Autodesk Inventor part; units mm, degrees
ref_plane "YZ Plane" through (0, 0, 0) normal (1, 0, 0) x (0, 1, 0)
ref_plane "XZ Plane" through (0, 0, 0) normal (0, 1, 0) x (-1, 0, 0)
ref_plane "XY Plane" through (0, 0, 0) normal (0, 0, 1) x (1, 0, 0)
sketch "Sketch1" plane through (0, 0, 0) normal (0, 1, 0) x (-1, 0, 0)
  circle A0 centre (4.364, -12.8492) radius 1.25
  line L0 (2.1213, -19.0919) -> (-8.4853, -8.4853)
  line L1 (10.6066, -10.6066) -> (0, 0)
  line L2 (0, 0) -> (-8.4853, -8.4853)
  circle A1 centre (-0.7071, -7.7782) radius 1.25
  line L3 (2.1213, -19.0919) -> (41.8977, -58.8682)
  line L4 (10.6066, -10.6066) -> (50.383, -50.383)
  arc A2 (41.8977, -58.8682) -> (50.383, -50.383) centre (55.8614, -64.3467) ccw
  circle A3 centre (62.579, -71.0642) radius 1.5
  circle A4 centre (49.1439, -57.6292) radius 1.5
  circle A5 centre (50.2046, -70.0036) radius 1.5
  circle A6 centre (61.5183, -58.6899) radius 1.5
  point P0 (0, 0)
  dimension "d3" = 3
  dimension "d4" = 3
  dimension "d5" = 3
  dimension "d6" = 3
extrude "Extrusion1" add sketch "Sketch1" along normal blind 3
sketch "Sketch2" plane through (0, 3, 0) normal (0, 1, 0) x (1, 0, 0)
  arc A0 (-41.8977, 58.8682) -> (-50.383, 50.383) centre (-55.8614, 64.3467) ccw
  circle A1 centre (-55.8614, 64.3467) radius 4
  point P0 (0, 0)
  dimension "d9" = 8
extrude "Extrusion2" cut sketch "Sketch2" against normal blind 3
properties part number "arm"
For this review, take the finished solid that the model builds, in its own axes (mm). Round coordinates to 2 decimals unless told otherwise and drop trailing zeros. Order: outer loops, then holes, each group sorted by start corner. A loop starts at its lowest first (then second) coordinate and runs counter-clockwise, first axis right, second up. Notation, with made-up numbers: (-20, 89) -> (-5, 89) arc R35 cw to (-5, 126) -> close; hole circle Ø3 at (59.25, 40). An arc over 180 degrees is marked (long way). Put each result on its own line as item: value.
Q1. Mouldability with a two-part tool opening along X and no side actions: class faces 1 (the cylindrical face through (0.13, 1.48, -6.67)), 2 (the flat face through (4, 1, -4)), 3 (the flat face through (-37, 3, -45)) as pulls with the +X half, pulls with the -X half, needs draft (parallel to the pull), parting line crosses it, or undercut.
Check result:
face 1: undercut
face 2: pulls with the +X half
face 3: needs draft
Q2. Insertion check: pin 1 Ø1.5 at (x, z) = (-4.36, -12.85) entering from +Y. The pin has a flat end and moves straight along its axis. Give the tip position at first contact, or say it passes through.
Check result:
pin 1: through
Q3. For probe 1 along Z at (x, y) = (-56, 0.25); probe 2 along Z at (x, y) = (-50, 2.8); probe 3 along Z at (x, y) = (-62, 0.75), list the stretches that pass through material, from the lowest coordinate up. Write a range as [from, to].
Check result:
probe 1: [-79.35, -68.34], [-60.35, -49.35]
probe 2: [-78.15, -71.49], [-68.52, -58.86], [-56.4, -50]
probe 3: [-78.03, -72.45], [-69.68, -60.11], [-57.27, -50.66]
Q4. Add section B-B on y = 1.6. Write out the cut boundary in (x, z), plus the area to 3 significant figures.
Check result:
outline: (-50.38, -50.38) arc R15 ccw (long way) to (-41.9, -58.87) -> (-2.12, -19.09) -> (8.49, -8.49) -> (0, 0) -> close; hole circle Ø3 at (-62.58, -71.06); hole circle Ø3 at (-61.52, -58.69); hole circle Ø8 at (-55.86, -64.35); hole circle Ø3 at (-50.2, -70); hole circle Ø3 at (-49.14, -57.63); hole circle Ø2.5 at (-4.36, -12.85); hole circle Ø2.5 at (0.71, -7.78)
area: 1,460 mm2
Q5. Add section C-C on x = -65. Write out the cut boundary in (y, z), plus the area to 3 significant figures.
Check result:
outline: (0, -76.24) -> (3, -76.24) -> (3, -52.45) -> (0, -52.45) -> close
area: 71.4 mm2
Q6. Add section D-D on z = -22. Write out the cut boundary in (x, y).
Check result:
outline: (-22, 0) -> (-5.03, 0) -> (-5.03, 3) -> (-22, 3) -> close
Q7. Add section A-A on x = -55.5. Write out the cut boundary in (y, z).
Check result:
outline: (0, -79.34) -> (3, -79.34) -> (3, -68.33) -> (0, -68.33) -> close; (0, -60.36) -> (3, -60.36) -> (3, -49.35) -> (0, -49.35) -> close
